from build123d import *

# Parameters (mm, degrees)
F0_R     = 25.527
F1_DEPTH = 25.4


with BuildPart() as f1:
    # F0 (on Top) → F1 (new body)
    with BuildSketch(Plane.XY):
        with BuildLine():
            ThreePointArc((50.799873, -0.113378), (50.799968, -0.056689), (50.8, 0))
            ThreePointArc((50.8, 0), (50.799968, 0.056689), (50.799873, 0.113378))
            ThreePointArc((50.799873, 0.113378), (46.168388, 4.15523), (50.003743, 8.959112))
            ThreePointArc((50.003743, 8.959112), (49.983623, 9.07069), (49.963254, 9.182224))
            ThreePointArc((49.963254, 9.182224), (44.684498, 12.332138), (47.600451, 17.743648))
            ThreePointArc((47.600451, 17.743648), (47.560731, 17.849841), (47.520775, 17.955945))
            ThreePointArc((47.520775, 17.955945), (41.764412, 20.112681), (43.667242, 25.957889))
            ThreePointArc((43.667242, 25.957889), (43.609199, 26.055283), (43.550939, 26.152548))
            ThreePointArc((43.550939, 26.152548), (37.501983, 27.246785), (38.330531, 33.337822))
            ThreePointArc((38.330531, 33.337822), (38.25603, 33.423287), (38.181339, 33.508586))
            ThreePointArc((38.181339, 33.508586), (32.034209, 33.505156), (31.761846, 39.64625))
            ThreePointArc((31.761846, 39.64625), (31.673282, 39.717039), (31.584561, 39.78763))
            ThreePointArc((31.584561, 39.78763), (25.53683, 38.686643), (24.172308, 44.680415))
            ThreePointArc((24.172308, 44.680415), (24.072528, 44.734253), (23.972628, 44.787868))
            ThreePointArc((23.972628, 44.787868), (18.218675, 42.62471), (15.805853, 48.278515))
            ThreePointArc((15.805853, 48.278515), (15.698063, 48.313671), (15.590195, 48.348586))
            ThreePointArc((15.590195, 48.348586), (10.314958, 45.192783), (6.931385, 50.324903))
            ThreePointArc((6.931385, 50.324903), (6.81905, 50.340248), (6.706681, 50.355342))
            ThreePointArc((6.706681, 50.355342), (2.079709, 46.308324), (-2.165864, 50.753808))
            ThreePointArc((-2.165864, 50.753808), (-2.279133, 50.748848), (-2.392392, 50.743635))
            ThreePointArc((-2.392392, 50.743635), (-2.378638, 50.54215), (-2.37405, 50.340248))
            ThreePointArc((-2.37405, 50.340248), (-6.423073, 45.912921), (-11.1935, 49.551444))
            ThreePointArc((-11.1935, 49.551444), (-11.304063, 49.526338), (-11.414571, 49.500986))
            ThreePointArc((-11.414571, 49.500986), (-11.293625, 48.912796), (-11.253063, 48.313671))
            ThreePointArc((-11.253063, 48.313671), (-14.906818, 43.939662), (-19.861368, 46.756455))
            ThreePointArc((-19.861368, 46.756455), (-19.965672, 46.712011), (-20.069876, 46.667334))
            ThreePointArc((-20.069876, 46.667334), (-19.739526, 45.725776), (-19.627528, 44.734253))
            ThreePointArc((-19.627528, 44.734253), (-22.892385, 40.448779), (-27.890875, 42.458675))
            ThreePointArc((-27.890875, 42.458675), (-27.985567, 42.396321), (-28.080119, 42.333756))
            ThreePointArc((-28.080119, 42.333756), (-27.446603, 41.092978), (-27.228282, 39.717039))
            ThreePointArc((-27.228282, 39.717039), (-30.113743, 35.554604), (-35.023946, 36.796239))
            ThreePointArc((-35.023946, 36.796239), (-35.105983, 36.717979), (-35.187844, 36.639536))
            ThreePointArc((-35.187844, 36.639536), (-34.169705, 35.172564), (-33.81103, 33.423287))
            ThreePointArc((-33.81103, 33.423287), (-36.329652, 29.417405), (-41.031319, 29.951141))
            ThreePointArc((-41.031319, 29.951141), (-41.098063, 29.859491), (-41.164603, 29.767692))
            ThreePointArc((-41.164603, 29.767692), (-39.696127, 28.163813), (-39.164199, 26.055283))
            ThreePointArc((-39.164199, 26.055283), (-41.331491, 22.238207), (-45.719912, 22.143389))
            ThreePointArc((-45.719912, 22.143389), (-45.769218, 22.041294), (-45.818297, 21.939089))
            ThreePointArc((-45.818297, 21.939089), (-43.85242, 20.300648), (-43.115731, 17.849841))
            ThreePointArc((-43.115731, 17.849841), (-44.950033, 14.252303), (-48.939029, 13.62393))
            ThreePointArc((-48.939029, 13.62393), (-48.969313, 13.514672), (-48.999354, 13.405346))
            ThreePointArc((-48.999354, 13.405346), (-46.509929, 11.844041), (-45.538623, 9.07069))
            ThreePointArc((-45.538623, 9.07069), (-47.060954, 5.721656), (-50.585205, 4.666587))
            ThreePointArc((-50.585205, 4.666587), (-50.595494, 4.553677), (-50.605531, 4.440744))
            ThreePointArc((-50.605531, 4.440744), (-47.588891, 3.073566), (-46.355, 0))
            ThreePointArc((-46.355, 0), (-47.588891, -3.073566), (-50.605531, -4.440744))
            ThreePointArc((-50.605531, -4.440744), (-50.595494, -4.553677), (-50.585205, -4.666587))
            ThreePointArc((-50.585205, -4.666587), (-47.060954, -5.721656), (-45.538623, -9.07069))
            ThreePointArc((-45.538623, -9.07069), (-46.509929, -11.844041), (-48.999354, -13.405346))
            ThreePointArc((-48.999354, -13.405346), (-48.969313, -13.514672), (-48.939029, -13.62393))
            ThreePointArc((-48.939029, -13.62393), (-44.950033, -14.252303), (-43.115731, -17.849841))
            ThreePointArc((-43.115731, -17.849841), (-43.85242, -20.300648), (-45.818297, -21.939089))
            ThreePointArc((-45.818297, -21.939089), (-45.769218, -22.041294), (-45.719912, -22.143389))
            ThreePointArc((-45.719912, -22.143389), (-41.331491, -22.238207), (-39.164199, -26.055283))
            ThreePointArc((-39.164199, -26.055283), (-39.696127, -28.163813), (-41.164603, -29.767692))
            ThreePointArc((-41.164603, -29.767692), (-41.098063, -29.859491), (-41.031319, -29.951141))
            ThreePointArc((-41.031319, -29.951141), (-36.329652, -29.417405), (-33.81103, -33.423287))
            ThreePointArc((-33.81103, -33.423287), (-34.169705, -35.172564), (-35.187844, -36.639536))
            ThreePointArc((-35.187844, -36.639536), (-35.105983, -36.717979), (-35.023946, -36.796239))
            ThreePointArc((-35.023946, -36.796239), (-30.113743, -35.554604), (-27.228282, -39.717039))
            ThreePointArc((-27.228282, -39.717039), (-27.446603, -41.092978), (-28.080119, -42.333756))
            ThreePointArc((-28.080119, -42.333756), (-27.985567, -42.396321), (-27.890875, -42.458675))
            ThreePointArc((-27.890875, -42.458675), (-22.892385, -40.448779), (-19.627528, -44.734253))
            ThreePointArc((-19.627528, -44.734253), (-19.739526, -45.725776), (-20.069876, -46.667334))
            ThreePointArc((-20.069876, -46.667334), (-19.965672, -46.712011), (-19.861368, -46.756455))
            ThreePointArc((-19.861368, -46.756455), (-14.906818, -43.939662), (-11.253063, -48.313671))
            ThreePointArc((-11.253063, -48.313671), (-11.293625, -48.912796), (-11.414571, -49.500986))
            ThreePointArc((-11.414571, -49.500986), (-11.304063, -49.526338), (-11.1935, -49.551444))
            ThreePointArc((-11.1935, -49.551444), (-6.423073, -45.912921), (-2.37405, -50.340248))
            ThreePointArc((-2.37405, -50.340248), (-2.378638, -50.54215), (-2.392392, -50.743635))
            ThreePointArc((-2.392392, -50.743635), (-2.279133, -50.748848), (-2.165864, -50.753808))
            ThreePointArc((-2.165864, -50.753808), (2.079709, -46.308324), (6.706681, -50.355342))
            ThreePointArc((6.706681, -50.355342), (6.81905, -50.340248), (6.931385, -50.324903))
            ThreePointArc((6.931385, -50.324903), (10.314958, -45.192783), (15.590195, -48.348586))
            ThreePointArc((15.590195, -48.348586), (15.698063, -48.313671), (15.805853, -48.278515))
            ThreePointArc((15.805853, -48.278515), (18.218675, -42.62471), (23.972628, -44.787868))
            ThreePointArc((23.972628, -44.787868), (24.072528, -44.734253), (24.172308, -44.680415))
            ThreePointArc((24.172308, -44.680415), (25.53683, -38.686643), (31.584561, -39.78763))
            ThreePointArc((31.584561, -39.78763), (31.673282, -39.717039), (31.761846, -39.64625))
            ThreePointArc((31.761846, -39.64625), (32.034209, -33.505156), (38.181339, -33.508586))
            ThreePointArc((38.181339, -33.508586), (38.25603, -33.423287), (38.330531, -33.337822))
            ThreePointArc((38.330531, -33.337822), (37.501983, -27.246785), (43.550939, -26.152548))
            ThreePointArc((43.550939, -26.152548), (43.609199, -26.055283), (43.667242, -25.957889))
            ThreePointArc((43.667242, -25.957889), (41.764412, -20.112681), (47.520775, -17.955945))
            ThreePointArc((47.520775, -17.955945), (47.560731, -17.849841), (47.600451, -17.743648))
            ThreePointArc((47.600451, -17.743648), (44.684498, -12.332138), (49.963254, -9.182224))
            ThreePointArc((49.963254, -9.182224), (49.983623, -9.07069), (50.003743, -8.959112))
            ThreePointArc((50.003743, -8.959112), (46.168388, -4.15523), (50.799873, -0.113378))
        make_face()
        Circle(F0_R, mode=Mode.SUBTRACT)
    extrude(amount=F1_DEPTH)


solid = f1.part
The model under review builds one solid part; all positions refer to its coordinate system, in mm. Give positions to 0.01 mm unless a question says otherwise; leave off trailing zeros. Order: outer loops, then holes, each group sorted by start corner. A loop starts at its lowest first (then second) coordinate and runs counter-clockwise, first axis right, second up. Notation, with made-up numbers: M -1.5,-11 L 6.5,-11 A19 ccw 6.5,10 Z; hole C 17.5,-16.5 d2. An arc over 180 degrees is marked long. Answer in a Markdown table with one row per item. Add a question column.
1. For pin 1 Ø1.5 at (y, z) = (-15.5, 9) entering from -X (3 decimals); pin 2 Ø2 at (y, z) = (-39, 16) entering from +X; pin 3 Ø1 at (y, z) = (-11.5, 16) entering from -X, all flat-tipped, find the tip position at first contact; note any pin that passes through.
2. To check wall thickness, follow line 1 along Y through (x, z) = (-41, 12); line 2 along X through (y, z) = (-15.5, 9.25); line 3 along Y through (x, z) = (0, 20.25). State the ranges of each line that lie inside material, in increasing order.
3. Add section A-A on y = -12. State the section outline as (x, z) points, plus the area to 3 significant figures.
4. Add section B-B on x = 0. State the section outline as (y, z) points, plus the area to 3 significant figures.
The answers:
| question | item | result |
|---|---|---|
| 1 | pin 1 | x = -44.375 |
| 1 | pin 2 | x = 31.76 |
| 1 | pin 3 | x = -46.64 |
| 2 | line 1 | -29.93 to -29.65, -22.46 to 22.46, 29.65 to 29.93 |
| 2 | line 2 | -43.79 to -20.28, 20.28 to 44.99 |
| 2 | line 3 | -46.93 to -25.53, 25.53 to 46.93 |
| 3 | outline | M -46.64,0 L -22.53,0 L -22.53,25.4 L -46.64,25.4 Z; M 22.53,0 L 44.79,0 L 44.79,25.4 L 22.53,25.4 Z |
| 3 | area | 1,180 mm2 |
| 4 | outline | M -46.93,0 L -25.53,0 L -25.53,25.4 L -46.93,25.4 Z; M 25.53,0 L 46.93,0 L 46.93,25.4 L 25.53,25.4 Z |
| 4 | area | 1,090 mm2 |
